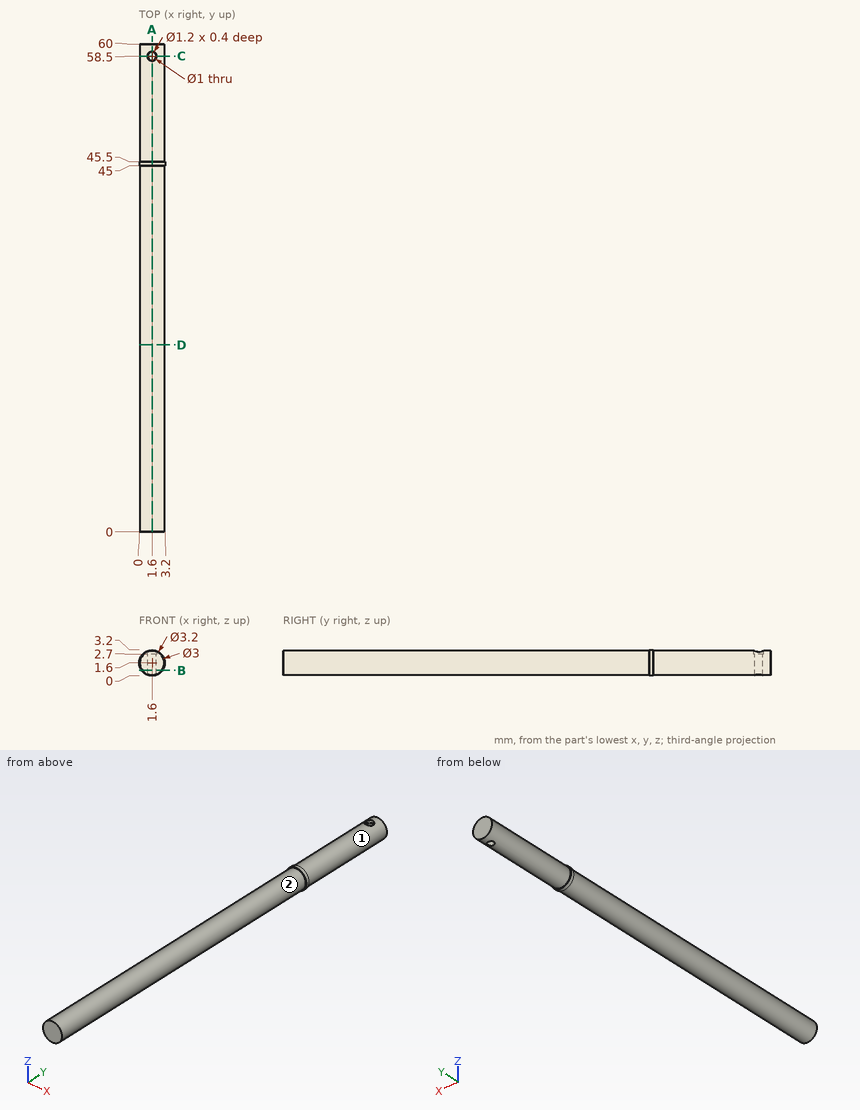
Can you work these out from the drawing? Everything is in mm from the part's minimum corner. A direction names the side the tool comes from. Round coordinates to 2 decimals unless told otherwise and drop trailing zeros. Order: outer loops, then holes, each group sorted by start corner. A loop starts at its lowest first (then second) coordinate and runs counter-clockwise, first axis right, second up.
(1) If I drill on L1, parallel to Y at x = 1.6, z = 3.05; L2, parallel to X at y = 27, z = 1.5; L3, parallel to X at y = 58.5, z = 2.85, over which ranges is the centre line in solid material (lowest first)?
Results are:
L1: y = 0 to 57.9, 59.1 to 60
L2: x = 0.1 to 3.1
L3: x = 0.77 to 1, 2.2 to 2.43
(2) If we section it at A-A (x = 1.6): Please give me the cut outline in (y, z), plus the area to 3 significant figures.
Results are:
outline: (0, 0.1) - (45, 0.1) - (45, 0) - (45.5, 0) - (45.5, 0.1) - (58, 0.1) - (58, 2.7) - (57.9, 2.7) - (57.9, 3.1) - (45.5, 3.1) - (45.5, 3.2) - (45, 3.2) - (45, 3.1) - (0, 3.1) - close; (59, 0.1) - (60, 0.1) - (60, 3.1) - (59.1, 3.1) - (59.1, 2.7) - (59, 2.7) - close
area: 177 mm2
(3) If we section it at C-C (y = 58.5): Please give me the cut outline in (x, z), plus the area to 3 significant figures.
Results are:
outline: (1, 2.7) - (1, 2.97) arc R1.5 ccw to (1.1, 0.19) - (1.1, 2.7) - close; (2.1, 0.19) arc R1.5 ccw to (2.2, 2.97) - (2.2, 2.7) - (2.1, 2.7) - close
area: 4.07 mm2
(4) On a 3-axis mill with a long thin cutter (end or side, diameter ignored), from which of +Z, -Z, +X, -X, +Y, -Y can I reach the whole of each face in a straight line? I mean the marked faces 1 and 2. Say none if no direction works.
Results are:
face 1: +Y
face 2: -Y
(5) If we section it at D-D (y = 23): Please give me the cut outline in (x, z).
Results are:
outline: circle Ø3 at (1.6, 1.6)
(6) I'm going to push a flat-ended pin straight in: pin 1 (1.5 mm diameter, centred on x = 2, y = 46.5, fed in from +Z). Where does the tip first touch, or does it pass through?
Results are:
pin 1: stops at z = 3.1
(7) If we section it at B-B (z = 0.7): Please give me the cut outline in (x, y), plus the area to 3 significant figures.
Results are:
outline: (0.28, 45) - (0.4, 45) - (0.4, 0) - (2.8, 0) - (2.8, 45) - (2.92, 45) - (2.92, 45.5) - (2.8, 45.5) - (2.8, 60) - (0.4, 60) - (0.4, 45.5) - (0.28, 45.5) - close; hole circle Ø1 at (1.6, 58.5)
area: 143 mm2
